Source: CAD feature listing. Evaluate the final solid. Frame: model axes, mm. Give positions to 0.01 mm unless a question says otherwise; leave off trailing zeros. Loops run counter-clockwise (first coordinate to the right, second up) from the corner with the lowest first, then second, coordinate; pieces in that order, holes last. Notation, with made-up numbers: (81.25, 74) -> (127.25, 74) arc R38 cw to (127.25, 112) -> close; hole circle Ø2 at (68.25, 59). An arc over 180 degrees is marked (long way). Answer as a JSON object with one key per item and string values. Group by question number.
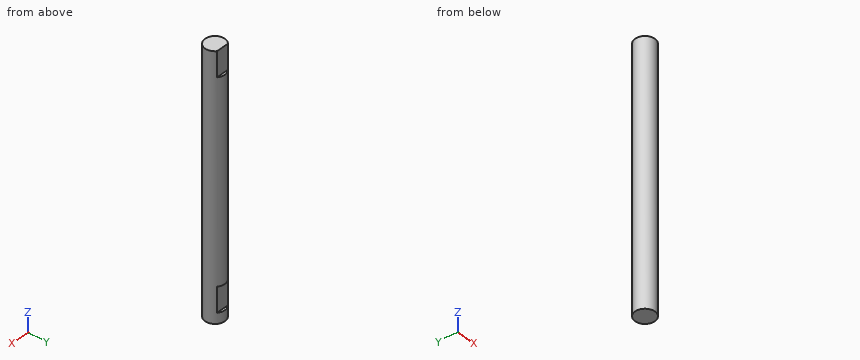
from build123d import *

# Parameters (mm, degrees)
SKETCH_1_R          = 4
EXTRUDE_1_DEPTH     = 104.25
CUT_EXTRUDE_1_DEPTH = 10


with BuildPart() as part:
    # 草图1 → 凸台-拉伸1 (new body)
    with BuildSketch(Plane.XY):
        with Locations((2.788805167, 15.198988159)):
            Circle(SKETCH_1_R)
    extrude(amount=EXTRUDE_1_DEPTH)

    # 草图2 → 切除-拉伸1 (cut)
    with BuildSketch(Plane.XY.offset(104.25)):
        Polygon((-1.211194833, 18.241175928), (6.788805167, 18.241175928), (6.788805167, 20.490551127), (-1.353486866, 20.490551127), (-1.451820208, 18.241175928), align=None)
    cut_extrude_1 = extrude(amount=-CUT_EXTRUDE_1_DEPTH, mode=Mode.SUBTRACT)

    # 镜向1: 切除-拉伸1 across plane
    add(cut_extrude_1.mirror(Plane.XY.offset(54.25)), mode=Mode.SUBTRACT)


solid = part.part
(1) Section query D-D on z = 49. Return the cut outline in (x, y).
(2) First-contact query: pin 1 (1.1 mm diameter, centred on x = 3, y = 19, fed in from +Z); pin 2 (2.5 mm diameter, centred on x = 3.5, z = 100, fed in from +Y); pin 3 (1 mm diameter, centred on y = 16, z = 86, fed in from -X). Flat tips, straight axial feed; report the tip coordinate or a pass-through.
(3) Section query A-A on x = 3.75. Return the cut outline in (y, z).
(4) Section query C-C on y = 13. Return the cut outline in (x, z), plus the area to 3 significant figures.
(5) Material intervals for line 1 (X direction, y = 15.5, z = 61); line 2 (Z direction, x = 2, y = 18.5); line 3 (Y direction, x = 3, z = 50.5), sorted ascending. Write a range as from..to.
(6) Section query B-B on z = 97. Return the cut outline in (x, y), plus the area to 3 significant figures.
Result:
{
 "1": {"outline": "circle Ø8 at (2.79, 15.2)"},
 "2": {"pin 1": "z = 94.25", "pin 2": "y = 18.24", "pin 3": "x = -1.2"},
 "3": {"outline": "(11.32, 0) -> (19.08, 0) -> (19.08, 4.25) -> (18.24, 4.25) -> (18.24, 14.25) -> (19.08, 14.25) -> (19.08, 94.25) -> (18.24, 94.25) -> (18.24, 104.25) -> (11.32, 104.25) -> close"},
 "4": {"outline": "(-0.55, 0) -> (6.13, 0) -> (6.13, 104.25) -> (-0.55, 104.25) -> close", "area": "697 mm²"},
 "5": {"line 1": "-1.2..6.78", "line 2": "0..4.25, 14.25..94.25", "line 3": "11.2..19.19"},
 "6": {"outline": "(0.19, 18.24) arc R4 ccw (long way) to (5.39, 18.24) -> close", "area": "46.9 mm²"}
}
